Answer from the drawing. Dimensions are ordinates in mm from the lowest x, y and z of the part. A direction names the side the tool comes from. Round coordinates to 2 decimals unless told otherwise and drop trailing zeros. Loops run counter-clockwise (first coordinate to the right, second up) from the corner with the lowest first, then second, coordinate; pieces in that order, holes last.
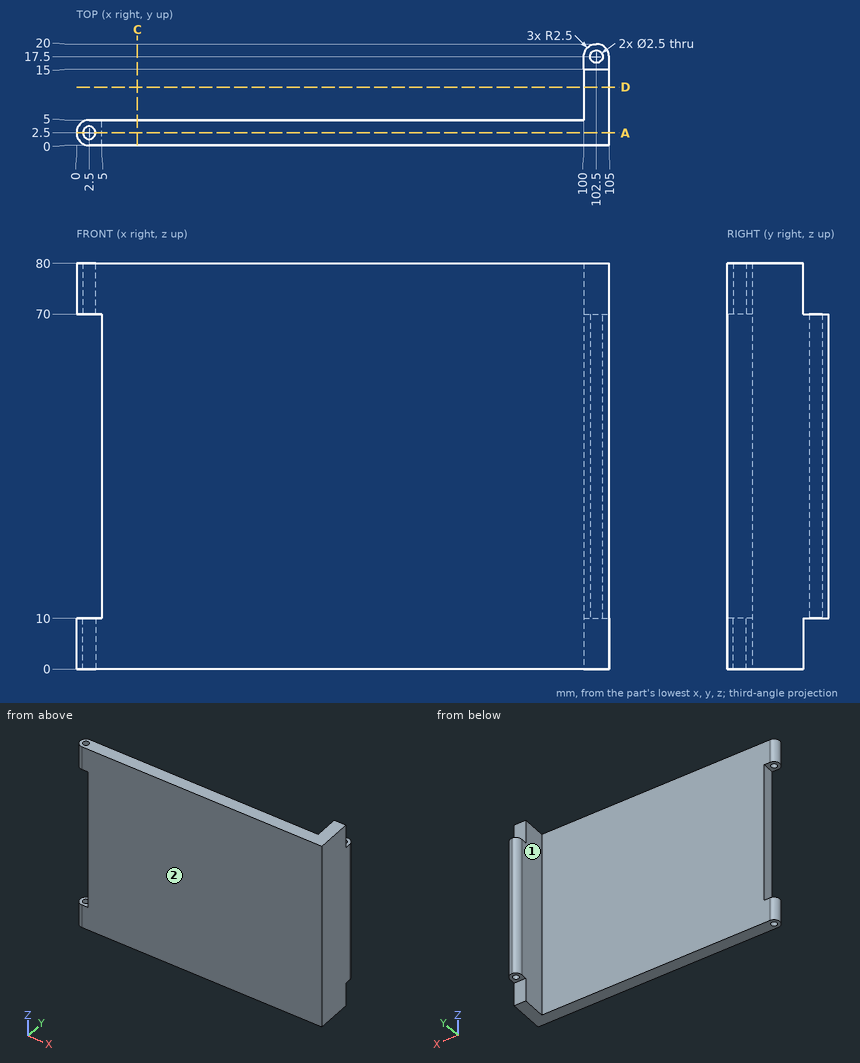
Item 1: Section D-D, the plane y = 11.5 is taken. Give the vertices of the cut face in (x, z), plus the area to 3 significant figures.
Item 2: Straight lines are drawn through the part: line 1 (X direction, y = 17.5, z = 39.5); line 2 (Y direction, x = 102.5, z = 48.5); line 3 (Y direction, x = 2.5, z = 7). For each, find the intervals that lie inside material, in ascending order.
Item 3: Section A-A, the plane y = 2.5 is taken. Give the vertices of the cut face in (x, z), plus the area to 3 significant figures.
Item 4: Each of these flat-tipped pins is pushed along its axis until it touches: P1, Ø5.5, axis at y = 2.5, z = 27.5, coming from the -X side; P2, Ø2.5, axis at x = 102.5, z = 3.5, coming from the +Y side; P3, Ø4, axis at x = 103, y = 18, coming from the +Z side. Where does it stop, or does it pass through?
Item 5: Section C-C, the plane x = 12 is taken. Give the vertices of the cut face in (y, z), plus the area to 3 significant figures.
Item 6: For the marked faces 1 and 2, determine the directions among +Z, -Z, +X, -X, +Y, -Y from which every point of the face is accessible in a straight line to the end or side of a thin tool.
Answer below:
1. outline: (100, 0) - (105, 0) - (105, 80) - (100, 80) - close
1. area: 400 mm2
2. line 1: x = 100 to 101.25, 103.75 to 105
2. line 2: y = 0 to 16.25, 18.75 to 20
2. line 3: y = 0 to 1.25, 3.75 to 5
3. outline: (0, 0) - (1.25, 0) - (1.25, 10) - (0, 10) - close; (0, 70) - (1.25, 70) - (1.25, 80) - (0, 80) - close; (3.75, 0) - (105, 0) - (105, 80) - (3.75, 80) - (3.75, 70) - (5, 70) - (5, 10) - (3.75, 10) - close
3. area: 8,050 mm2
4. P1: stops at x = 5
4. P2: stops at y = 15
4. P3: stops at z = 70
5. outline: (0, 0) - (5, 0) - (5, 80) - (0, 80) - close
5. area: 400 mm2
6. face 1: +Z, -Z, -X, +Y
6. face 2: +Z, -Z, +X, -X, -Y
